Autodesk Inventor part; units mm, degrees
ref_plane "YZ Plane" through (0, 0, 0) normal (1, 0, 0) x (0, 1, 0)
ref_plane "XZ Plane" through (0, 0, 0) normal (0, 1, 0) x (-1, 0, 0)
ref_plane "XY Plane" through (0, 0, 0) normal (0, 0, 1) x (1, 0, 0)
sketch "Sketch1" plane through (0, 0, 0) normal (0, 1, 0) x (-1, 0, 0)
  line L0 (-45, 35) -> (45, 35)
  line L1 (45, 35) -> (45, -35)
  line L2 (45, -35) -> (-45, -35)
  line L3 (-45, -35) -> (-45, 35)
  line L4 (-45, 35) -> (45, -35) construction
  line L5 (45, 35) -> (-45, -35) construction
  line L6 (-48, 38) -> (48, 38)
  line L7 (48, 38) -> (48, -38)
  line L8 (48, -38) -> (-48, -38)
  line L9 (-48, -38) -> (-48, 38)
  line L10 (-48, 38) -> (48, -38) construction
  line L11 (48, 38) -> (-48, -38) construction
  line L12 (48, 38) -> (58, 38)
  line L13 (58, 38) -> (58, -38)
  line L14 (58, -38) -> (48, -38)
  line L15 (48, -38) -> (48, 38)
  line L16 (-48, 38) -> (-58, 38)
  line L17 (-58, 38) -> (-58, -38)
  line L18 (-58, -38) -> (-48, -38)
  line L19 (-48, -38) -> (-48, 38)
  line L20 (54, -19) -> (54, 19)
  line L21 (54, -19) -> (92, -19) construction
  circle A0 centre (54, 19) radius 1.5
  circle A1 centre (54, -19) radius 1.5
  line L22 (-54, -19) -> (-54, 19)
  circle A2 centre (-54, 19) radius 1.5
  circle A3 centre (-54, -19) radius 1.5
  line L23 (58, 0) -> (54, 0)
  line L24 (-58, 0) -> (-54, 0)
  point P0 (0, 0)
  point P1 (54, 0)
  dimension "d0" = 90
  dimension "d1" = 70
  dimension "d2" = 96
  dimension "d3" = 76
  dimension "d4" = 10
  dimension "d5" = 76
  dimension "d6" = 10
  dimension "d7" = 76
  dimension "d8" = 38
  dimension "d9" = 90
  dimension "d10" = 3
  dimension "d11" = 3
  dimension "d12" = 3
  dimension "d13" = 3
  dimension "d23" = 4
  dimension "d24" = 4
extrude "Extrusion1" add sketch "Sketch1" against normal blind 20 contours L6 L7 L8 L9
extrude "Extrusion2" add sketch "Sketch1" against normal blind 2 contours L9 L18 L17 L16 | L12 L13 L14 L7
sketch "Sketch2" plane through (0, -20, 0) normal (0, -1, 0) x (1, 0, 0)
  line L0 (-48, -38) -> (48, -38)
  line L1 (-48, 38) -> (48, 38)
  line L2 (48, 38) -> (48, -38)
  line L3 (48, -38) -> (-48, -38)
  line L4 (-48, -38) -> (-48, 38)
  line L5 (-48, 38) -> (48, -38) construction
  line L6 (48, 38) -> (-48, -38) construction
  point P0 (0, 0)
extrude "Extrusion3" add sketch "Sketch2" along normal blind 2
fillet "Fillet1" radius 5 8 edges at (48, -12, -38) (-48, -12, -38) (48, -12, 38) (-48, -12, 38) (-58, -1, 38) (-58, -1, -38) (58, -1, -38) (58, -1, 38)
fillet "Fillet2" radius 1 1 edges at (48, -2, 0)
fillet "Fillet3" radius 3 8 edges at (-46.5355, -22, 36.5355) (-48, -22, 0) (-46.5355, -22, -36.5355) (0, -22, -38) (46.5355, -22, -36.5355) (48, -22, 0) (46.5355, -22, 36.5355) (0, -22, 38)
properties part number "battary holder"
CAD build for the part. Positions are in the model's coordinates, mm. A direction names the side the tool comes from. Give positions to 0.01 mm unless a question says otherwise; leave off trailing zeros. Write each loop counter-clockwise with the first axis right and the second up, starting at its lowest first coordinate (ties: lowest second). Pieces come first, ordered by that corner, then holes. Notation, with made-up numbers: (-1, 38) - (3, 38) arc R24 ccw to (3, 54) - close; hole circle Ø10 at (33.25, -14). An arc over 180 degrees is marked (long way). Answer as CSV lines item,"result".
Q1. Band-saw the part on C-C (x = 7.5). Give the cut face in (y, z).
Result set:
outline,"(-22, -35) arc R3 ccw to (-19, -38) - (0, -38) - (0, -35) - (-20, -35) - (-20, 35) - (0, 35) - (0, 38) - (-19, 38) arc R3 ccw to (-22, 35) - close"
Q2. Flat gauge pins, fed straight in: pin 1 Ø12 at (x, z) = (-1, -17.5) entering from +Y; pin 2 Ø5 at (y, z) = (-12, 6) entering from -X; pin 3 Ø13 at (y, z) = (-14.5, 15.5) entering from +X. Where does each tip first touch, or does it go through?
Result set:
pin 1,"y = -20"
pin 2,"x = -48"
pin 3,"x = 48"
Q3. Band-saw the part on B-B (y = -13.25). Give the cut face in (x, z).
Result set:
outline,"(-48, -33) arc R5 ccw to (-43, -38) - (43, -38) arc R5 ccw to (48, -33) - (48, 33) arc R5 ccw to (43, 38) - (-43, 38) arc R5 ccw to (-48, 33) - close; hole (-45, -35) - (45, -35) - (45, 35) - (-45, 35) - close"
Q4. Band-saw the part on A-A (z = 19). Give the cut face in (x, y), and give its area (3 significant figures).
Result set:
outline,"(-58, -2) - (-55.5, -2) - (-55.5, 0) - (-58, 0) - close; (-52.5, -2) - (-48, -2) - (-48, -19) arc R3 ccw to (-45, -22) - (45, -22) arc R3 ccw to (48, -19) - (48, -3) arc R1 cw to (49, -2) - (52.5, -2) - (52.5, 0) - (45, 0) - (45, -20) - (-45, -20) - (-45, 0) - (-52.5, 0) - close; (55.5, -2) - (58, -2) - (58, 0) - (55.5, 0) - close"
area,"336 mm²"
Q5. Band-saw the part on D-D (z = -16). Give the cut face in (x, y), and give its area (3 significant figures).
Result set:
outline,"(-58, -2) - (-48, -2) - (-48, -19) arc R3 ccw to (-45, -22) - (45, -22) arc R3 ccw to (48, -19) - (48, -3) arc R1 cw to (49, -2) - (58, -2) - (58, 0) - (45, 0) - (45, -20) - (-45, -20) - (-45, 0) - (-58, 0) - close"
area,"348 mm²"
Q6. 3-axis set-ups, long thin cutter, end or side, ignore diameter. For faces 1 (the face through (46, -11, 37)), 2 (the face through (-0.6, -21.1, -37.14)), 3 (the face through (46, -11, -37)), 4 (the face through (-1, -10, -35)): which of +Z, -Z, +X, -X, +Y, -Y reach the whole face in a straight line?
Result set:
face 1,"+Z, +X, -Y"
face 2,"-Z, +X, -X, -Y"
face 3,"-Z, +X, -Y"
face 4,"+Y"
Q7. Pull direction X, two halves, no side cores. Call faces 5 (the face through (54.195, -0.986, -17.513)), 6 (the face through (45, -10, 0)), 7 (the face through (0, 0, 37)), 8 (the face through (-48, -10, 0)): released by +X, released by -X, zero draft, split by the parting line, or undercut.
Result set:
face 5,"undercut"
face 6,"undercut"
face 7,"zero draft"
face 8,"released by -X"
Q8. Drill centre lines: line 1 (X direction, y = -1.5, z = 19); line 2 (Z direction, x = 31.5, y = -16); line 3 (X direction, y = -11.75, z = 23). Where is each one in solid material? Low to high. Write a range as from..to.
Result set:
line 1,"-58..-55.5, -52.5..-45, 45..52.5, 55.5..58"
line 2,"-38..-35, 35..38"
line 3,"-48..-45, 45..48"
